Model file for the job. Use its own axes, mm. Give positions to 0.01 mm unless a question says otherwise; leave off trailing zeros. Loops run counter-clockwise (first coordinate to the right, second up) from the corner with the lowest first, then second, coordinate; pieces in that order, holes last. Notation, with made-up numbers: M 46,-14 L 63,-14 A14 ccw 63,2 Z; hole C 16,21.25 d5. An arc over 180 degrees is marked long. Answer in a Markdown table with one row per item.
Autodesk Inventor part; units mm, degrees
ref_plane "YZ Plane" through (0, 0, 0) normal (1, 0, 0) x (0, 1, 0)
ref_plane "XZ Plane" through (0, 0, 0) normal (0, 1, 0) x (-1, 0, 0)
ref_plane "XY Plane" through (0, 0, 0) normal (0, 0, 1) x (1, 0, 0)
sketch "Sketch1" plane through (0, 0, 0) normal (0, 1, 0) x (-1, 0, 0)
  circle A0 centre (0, 0) radius 200
  line L0 (0, 0) -> (0, -19)
  line L1 (0, 0) -> (0, -200)
  line L2 (0, -200) -> (0, -185)
  line L3 (0, -185) -> (-40, -185)
  line L4 (-40, -185) -> (40, -185)
  line L5 (40, -185) -> (40, -155)
  line L6 (40, -155) -> (-40, -155)
  line L7 (-40, -155) -> (-40, -185)
  line L8 (0, -185) -> (0, -155)
  line L9 (0, -155) -> (0, -170)
  line L10 (0, -170) -> (0, -178.5)
  line L11 (0, -178.5) -> (0, -162.5)
  line L12 (0, -178.5) -> (0, -161.5)
  line L13 (0, -178.5) -> (0, -152.5)
  line L14 (0, -152.5) -> (0, -100.5)
  line L15 (0, -100.5) -> (0, -111.5)
  line L16 (0, -111.5) -> (0, -141.5)
  line L17 (0, -111.5) -> (62.5795, -111.5)
  line L18 (62.5795, -111.5) -> (-81.3818, -111.5)
  line L19 (0, -141.5) -> (67.2407, -141.5)
  line L20 (67.2407, -141.5) -> (-91.5277, -141.5)
  line L21 (0, -111.5) -> (19.187, -111.5)
  line L22 (19.187, -111.5) -> (-27.813, -111.5)
  line L23 (-27.813, -111.5) -> (-27.813, -148.582)
  line L24 (19.187, -111.5) -> (19.187, -155)
  circle A1 centre (19.187, -111.5) radius 2
  circle A2 centre (19.187, -141.5) radius 2
  circle A3 centre (-27.813, -111.5) radius 2
  circle A4 centre (-27.813, -141.5) radius 2
  line L25 (0, 0) -> (124.6952, 0)
  circle A5 centre (0, 0) radius 1
  circle A6 centre (-154.7094, 0) radius 1
  circle A7 centre (178.175, 0) radius 1
  line L26 (0, 185) -> (-40, 185)
  line L27 (-40, 185) -> (40, 185)
  line L28 (40, 185) -> (40, 155)
  line L29 (40, 155) -> (-40, 155)
  line L30 (-40, 155) -> (-40, 185)
  line L31 (0, 185) -> (0, 155)
  line L32 (0, 155) -> (0, 170)
  line L33 (0, 170) -> (0, 178.5)
  line L34 (0, 178.5) -> (0, 162.5)
  line L35 (0, 178.5) -> (0, 161.5)
  line L36 (0, 178.5) -> (0, 152.5)
  circle A8 centre (-19.187, 111.5) radius 2
  circle A9 centre (-19.187, 141.5) radius 2
  line L37 (27.813, 141.5) -> (-19.187, 141.5)
  line L38 (-19.187, 111.5) -> (27.813, 111.5)
  circle A10 centre (27.813, 111.5) radius 2
  circle A11 centre (27.813, 141.5) radius 2
  line L39 (27.813, 141.5) -> (27.813, 111.5)
  line L40 (-19.187, 141.5) -> (-19.187, 111.5)
  line L41 (0, 0) -> (0, 200)
  line L42 (0, -100.5) -> (0, 0)
  line L43 (0, 0) -> (0, 111.5)
  dimension "d0" = 400
  dimension "d2" = 15
  dimension "d3" = 40
  dimension "d4" = 80
  dimension "d5" = 30
  dimension "d6" = 80
  dimension "d7" = 8.5
  dimension "d8" = 17
  dimension "d9" = 26
  dimension "d10" = 52
  dimension "d15" = 4
  dimension "d16" = 4
  dimension "d17" = 4
  dimension "d18" = 4
  dimension "d21" = 2
  dimension "d22" = 2
  dimension "d23" = 2
  dimension "d35" = 47
  dimension "d36" = 30
  dimension "d37" = 19.187
  dimension "d38" = 11
  dimension "d39" = 4
  dimension "d40" = 47
  dimension "d41" = 30
  dimension "d42" = 111.5
  dimension "d43" = 19.187
extrude "Extrusion1" add sketch "Sketch1" along normal blind 6 contours A0 L1 L4 L5 L6 L24 A2 A1 L17 L0 A5 L41 L38 A10 L39 A11 L37 L36 L29 L28 L27 | L41 L26 L30 L29 L36 L37 A9 L40 A8 L38 A5 L0 L1 L18 A3 L23 A4 L20 L6 L7 L3 A0 | L1 L19 A2 L24 L6 | L41 L38 A8 L40 A9 L37 | L37 A11 L39 A10 L38 L41 | L20 A4 L23 A3 L18 L1 | L1 L17 A1 L24 A2 L19 | A6 | A7
sketch "Sketch2" plane through (0, 6, 0) normal (0, 1, 0) x (1, 0, 0)
  circle A0 centre (0, 0) radius 1
  line L0 (0, 0) -> (233.037, 233.037)
  line L1 (0, 0) -> (329.564, 0) construction
  line L2 (0, 0) -> (120.2082, 120.2082)
  circle A1 centre (120.2082, 120.2082) radius 1
  dimension "d24" = 45
  dimension "d25" = 170
  dimension "d26" = 2
extrude "Extrusion2" cut sketch "Sketch2" against normal blind 6 contours A1 L0 | L0 A1
pattern_circular "Circular Pattern1" count 8 over 360 about axis through (0, -10, 0) along (0, -1, 0) of "Extrusion2"
sketch "Sketch3" plane through (0, 6, 0) normal (0, 1, 0) x (1, 0, 0)
  circle A0 centre (0, 0) radius 1
  line L0 (0, 0) -> (200, 0)
  circle A1 centre (0, 0) radius 200
  line L1 (0, 0) -> (0, 398.337)
  line L2 (0, 398.337) -> (0, -304.2315)
  line L3 (0, 0) -> (-272.9704, 0)
  line L4 (200, 0) -> (174.2263, 0)
  line L5 (174.2263, 0) -> (174.2263, 12)
  line L6 (174.2263, 12) -> (127.2263, 12)
  line L7 (127.2263, 12) -> (127.2263, -12)
  line L8 (127.2263, -12) -> (174.2263, -12)
  line L9 (174.2263, -12) -> (174.2263, 12)
  circle A2 centre (127.2263, -12) radius 1.5
  circle A3 centre (127.2263, 12) radius 1.5
  circle A4 centre (174.2263, -12) radius 1.5
  circle A5 centre (174.2263, 12) radius 1.5
  dimension "d44" = 12
  dimension "d45" = 47
  dimension "d46" = 24
  dimension "d47" = 3
  dimension "d48" = 3
  dimension "d49" = 3
  dimension "d50" = 3
extrude "Extrusion3" cut sketch "Sketch3" against normal blind 6 contours A3 L6 L7 | L7 L6 A3 | A2 L8 L7 | L7 L8 A2 | A5 L6 L5 | L5 L6 A5 | A4 L8 L9 | L9 L8 A4
sketch "Sketch5" plane through (0, 6, 0) normal (0, 1, 0) x (1, 0, 0)
  circle A0 centre (0, 0) radius 200
  line L0 (200, 0) -> (183, 0)
  line L1 (183, 0) -> (183, 10)
  line L2 (183, 10) -> (183, 0)
  line L3 (183, 0) -> (183, -10)
  circle A1 centre (183, -10) radius 1.5
  circle A2 centre (183, 10) radius 1.5
  dimension "d53" = 17
  dimension "d54" = 10
  dimension "d55" = 10
  dimension "d56" = 10
  dimension "d57" = 3
  dimension "d58" = 3
extrude "Extrusion4" cut sketch "Sketch5" against normal blind 6 contours A1 | A2
pattern_circular "Circular Pattern2" count 2 over 45 about axis through (0, -10, 0) along (0, 1, 0) of "Extrusion4"
pattern_circular "Circular Pattern3" count 2 over 45 about axis through (0, -10, 0) along (0, -1, 0) of "Extrusion4"
sketch "Sketch6" plane through (0, 6, 0) normal (0, 1, 0) x (1, 0, 0)
  circle A0 centre (0, 0) radius 1
  line L0 (0, 0) -> (0, -130)
  line L1 (-40, -155) -> (40, -155)
  line L2 (0, -130) -> (0, 130)
  line L3 (100.075, -103.9398) -> (109.075, -103.9398)
  line L4 (109.075, -103.9398) -> (109.075, 102.0602)
  line L5 (109.075, 102.0602) -> (100.075, 102.0602)
  line L6 (100.075, 102.0602) -> (100.075, -103.9398)
  line L7 (100.075, -103.9398) -> (109.075, 102.0602) construction
  line L8 (109.075, -103.9398) -> (100.075, 102.0602) construction
  line L9 (100.075, 102.0602) -> (70.075, 102.0602)
  line L10 (70.075, 102.0602) -> (70.075, 57.0602)
  line L11 (70.075, 57.0602) -> (94.075, 57.0602)
  line L12 (94.075, 57.0602) -> (33.1028, 57.0602)
  line L13 (33.1028, 57.0602) -> (33.1028, -101.9398)
  line L14 (33.1028, -101.9398) -> (94.075, -101.9398)
  line L15 (94.075, -101.9398) -> (94.075, 57.0602)
  line L16 (0, -155) -> (0, -85)
  line L17 (0, -85) -> (-56.011, -85)
  line L18 (-56.011, -85) -> (54.9913, -85)
  line L19 (40, 155) -> (-40, 155)
  line L20 (0, 155) -> (0, 85)
  line L21 (0, 85) -> (-43.3575, 85)
  line L22 (-43.3575, 85) -> (43.7057, 85)
  line L23 (-50, -130) -> (50, -130)
  line L24 (50, -130) -> (50, 130)
  line L25 (50, 130) -> (-50, 130)
  line L26 (-50, 130) -> (-50, -130)
  circle A1 centre (0, 0) radius 1
  line L27 (-50, -130) -> (50, 130) construction
  line L28 (50, -130) -> (-50, 130) construction
  circle A2 centre (-50, -130) radius 2.5
  circle A3 centre (-50, 130) radius 2.5
  circle A4 centre (50, 130) radius 2.5
  circle A5 centre (50, -130) radius 2.5
  dimension "d68" = 130
  dimension "d69" = 260
  dimension "d70" = 9
  dimension "d71" = 206
  dimension "d73" = 30
  dimension "d74" = 45
  dimension "d75" = 70
  dimension "d76" = 70
  dimension "d79" = 100
  dimension "d80" = 260
  dimension "d81" = 5
  dimension "d82" = 5
  dimension "d83" = 5
  dimension "d84" = 5
extrude "Extrusion5" cut sketch "Sketch6" against normal blind 9 contours A0 L0 L2 | L2 L0 A0 | L5 L4 L3 L6 | A3 L26 L25 | L25 L26 A3 | A4 L24 L25 | L25 L24 A4 | A2 L26 L23 | L23 L26 A2 | A5 L24 L23 | L23 L24 A5
properties part number "Robot_base" material "Birch"
(1) Flat gauge pins, fed straight in: P1, Ø2, axis at y = 5, z = -51, coming from the +X side; P2, Ø1.8, axis at y = 3.5, z = 174.5, coming from the +X side; P3, Ø1, axis at y = 1, z = -82.5, coming from the -X side. Where does each tip first touch, or does it go through?
Established:
| item | result |
|---|---|
| P1 | stops at x = 193.65 |
| P2 | stops at x = 99.31 |
| P3 | stops at x = -182.42 |
(2) Saw through at B-B, the plane y = 2.5. Count the separate pieces of the cut face and the enclosed holes in it, and give its area (3 significant figures).
Established:
| item | result |
|---|---|
| separate pieces | 1 |
| enclosed holes | 32 |
| area | 119,000 mm2 |
(3) Saw through at A-A, the plane z = 32. Give the cut face in (x, y) (3 decimals), and give its area (3 significant figures).
Established:
| item | result |
|---|---|
| outline | M -197.423,0 L 100.075,0 L 100.075,6 L -197.423,6 Z; M 109.075,0 L 197.423,0 L 197.423,6 L 109.075,6 Z |
| area | 2,320 mm2 |
(4) Wall check: L1, parallel to X at y = 4.15, z = 0 (3 decimals); L2, parallel to Z at x = 123, y = 4.45; L3, parallel to Z at x = -21, y = 0.75. Give the ranges that are in metal, low to high.
Established:
| item | result |
|---|---|
| L1 | x = -200 to -171, -169 to -1, 1 to 100.075, 109.075 to 169, 171 to 200 |
| L2 | z = -157.71 to -137.81, -135.13 to 135.13, 137.81 to 157.71 |
| L3 | z = -198.89 to -185, -155 to -142.34, -140.66 to -112.34, -110.66 to 155, 185 to 198.89 |
(5) Saw through at D-D, the plane x = -148.5. Give the cut face in (y, z), and give its area (3 significant figures).
Established:
| item | result |
|---|---|
| outline | M 0,-133.97 L 6,-133.97 L 6,133.97 L 0,133.97 Z |
| area | 1,610 mm2 |
(6) Saw through at C-C, the plane x = 64. Give the cut face in (y, z), and give its area (3 significant figures).
Established:
| item | result |
|---|---|
| outline | M 0,-189.48 L 6,-189.48 L 6,189.48 L 0,189.48 Z |
| area | 2,270 mm2 |
